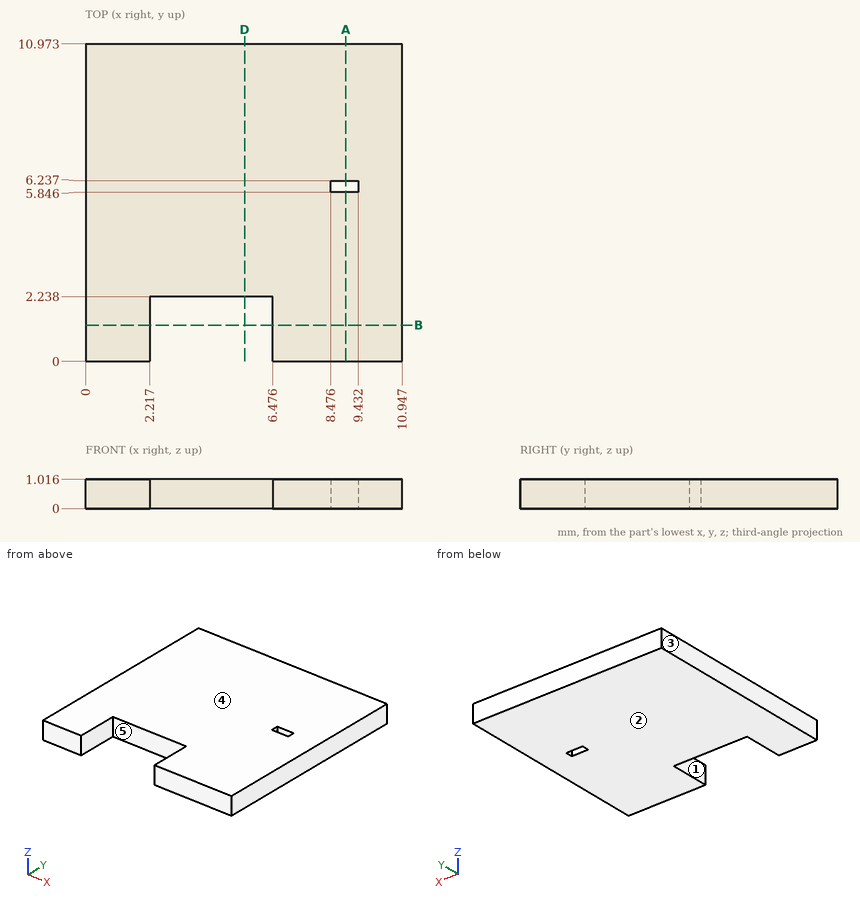
For this review, use the dimensioned drawing (mm, ordinates from the lowest corner) and the shaded views. A direction names the side the tool comes from. Give positions to 0.01 mm unless a question says otherwise; leave off trailing zeros. Order: outer loops, then holes, each group sorted by start corner. A loop starts at its lowest first (then second) coordinate and runs counter-clockwise, first axis right, second up.
1) Wall thickness on line 1 (Y direction, x = 9, z = 0.15); line 2 (X direction, y = 2, z = 0.4); line 3 (Y direction, x = 3.5, z = 0.45): over which ranges is each line inside the solid? List them lowest first.
2) Take a section at A-A (x = 9). Give the boundary of the cut face in (y, z).
3) For the marked faces 1 and 2, list the 3-axis set-ups (+Z, -Z, +X, -X, +Y, -Y) from which the entire face can be reached by the end or side of a thin tool; tool diameter is ignored.
4) Take a section at B-B (y = 1.25). Give the boundary of the cut face in (x, z).
5) Take a section at D-D (x = 5.5). Give the boundary of the cut face in (y, z).
6) The part is to be moulded in two halves that separate along X. For the marked faces 3, 4 and 5, say which applies: released by +X, released by -X, zero draft, split by the parting line, or undercut.
Derived:
1. line 1: y = 0 to 5.85, 6.24 to 10.97
1. line 2: x = 0 to 2.22, 6.48 to 10.95
1. line 3: y = 2.24 to 10.97
2. outline: (0, 0) - (5.85, 0) - (5.85, 1.02) - (0, 1.02) - close; (6.24, 0) - (10.97, 0) - (10.97, 1.02) - (6.24, 1.02) - close
3. face 1: +Z, -Z, -Y
3. face 2: -Z, +X, -X, +Y, -Y
4. outline: (0, 0) - (2.22, 0) - (2.22, 1.02) - (0, 1.02) - close; (6.48, 0) - (10.95, 0) - (10.95, 1.02) - (6.48, 1.02) - close
5. outline: (2.24, 0) - (10.97, 0) - (10.97, 1.02) - (2.24, 1.02) - close
6. face 3: released by -X
6. face 4: zero draft
6. face 5: undercut
